CAD build for the part. Positions are in the model's coordinates, mm. A direction names the side the tool comes from. Coordinates: 2 decimals unless noted, no trailing zeros. Loops run counter-clockwise (first coordinate to the right, second up) from the corner with the lowest first, then second, coordinate; pieces in that order, holes last. Notation, with made-up numbers: (70, 34) -> (105, 34) arc R8 ccw to (105, 41) -> close; hole circle Ø4 at (4, 17.5). An arc over 180 degrees is marked (long way). Write each question's results on one line, items separated by ' | '.
```python
from build123d import *

# Parameters (mm, degrees)
SKETCH1_W                     = 60
SKETCH1_H                     = 120
BASE_FLANGE1_DEPTH            = 1.5
CUT_EXTRUDE1_DEPTH            = 10
BREAK_CORNER1_START           = -1.5
BREAK_CORNER1_DEPTH           = 1.5
EDGE_FLANGE1_STRIP_W          = 8
EDGE_FLANGE1_STRIP_H          = 1.5
EDGE_FLANGE1_STRIP_CUT_DEPTH  = 20
EDGE_FLANGE1_RELIEF_W         = 9.5
EDGE_FLANGE1_RELIEF_H         = 1.5
EDGE_FLANGE1_RELIEF_CUT_DEPTH = 1.5
EDGE_FLANGE1_DEPTH            = 20
SKETCH10_R                    = 4
CUT_EXTRUDE2_DEPTH            = 10
MIRROR2_COPY_1_SKETCH_W       = 8
MIRROR2_COPY_1_SKETCH_H       = 1.5
MIRROR2_COPY_1_DEPTH          = 20
MIRROR2_COPY_2_SKETCH_W       = 9.5
MIRROR2_COPY_2_SKETCH_H       = 1.5
MIRROR2_COPY_2_DEPTH          = 1.5
MIRROR2_COPY_3_DEPTH          = 20
MIRROR2_COPY_4_SKETCH_R       = 4
MIRROR2_COPY_4_DEPTH          = 10
BREAK_CORNER2_START           = -30
BREAK_CORNER2_DEPTH           = 60


# Read off the part's stored shape, not the designer's step: Break-Corner1, Break-Corner2
# Sheet-metal steps are written as plain solids
with BuildPart() as part:
    # Sketch1 → Base-Flange1 (new body)
    with BuildSketch(Plane(origin=(0, 0, 0), x_dir=(1, 0, 0), z_dir=(0, 1, 0))):
        Rectangle(SKETCH1_W, SKETCH1_H)
    extrude(amount=-BASE_FLANGE1_DEPTH)

    # Sketch6 → Cut-Extrude1 (cut)
    with BuildSketch(Plane(origin=(0, 0, 0), x_dir=(1, 0, 0), z_dir=(0, 1, 0))):
        with BuildLine():
            Line((18, 30), (18, -30))
            ThreePointArc((18, -30), (0, -48), (-18, -30))
            Line((-18, -30), (-18, 30))
            ThreePointArc((-18, 30), (0, 48), (18, 30))
        make_face()
    extrude(amount=-CUT_EXTRUDE1_DEPTH, mode=Mode.SUBTRACT)

    # Break-Corner1 outline → Break-Corner1 (cut)
    with BuildSketch(Plane(origin=(0, 0, 0), x_dir=(1, 0, 0), z_dir=(0, 1, 0)).offset(BREAK_CORNER1_START)):
        with BuildLine():
            ThreePointArc((30, -50), (27.071067812, -57.071067812), (20, -60))
            Line((20, -60), (30, -60))
            Line((30, -60), (30, -50))
        make_face()
        with BuildLine():
            Line((-30, -60), (-20, -60))
            ThreePointArc((-20, -60), (-27.071067812, -57.071067812), (-30, -50))
            Line((-30, -50), (-30, -60))
        make_face()
        with BuildLine():
            ThreePointArc((20, 60), (27.071067812, 57.071067812), (30, 50))
            Line((30, 50), (30, 60))
            Line((30, 60), (20, 60))
        make_face()
        with BuildLine():
            Line((-30, 60), (-30, 50))
            ThreePointArc((-30, 50), (-27.071067812, 57.071067812), (-20, 60))
            Line((-20, 60), (-30, 60))
        make_face()
    extrude(amount=BREAK_CORNER1_DEPTH, mode=Mode.SUBTRACT)

    # Edge-Flange1 strip (across the edge) → Edge-Flange1 strip cut (cut)
    with BuildSketch(Plane(origin=(30, -1.5, 25), x_dir=(-1, 0, 0), z_dir=(0, 0, 1))):
        with Locations((-1.5, -0.75)):
            Rectangle(EDGE_FLANGE1_STRIP_W, EDGE_FLANGE1_STRIP_H)
    edge_flange1_strip_cut = extrude(amount=EDGE_FLANGE1_STRIP_CUT_DEPTH, mode=Mode.SUBTRACT)

    # Edge-Flange1 relief (on the sheet) → Edge-Flange1 relief cut (cut)
    with BuildSketch(Plane(origin=(27.5, -1.5, 25), x_dir=(-1, 0, 0), z_dir=(0, -1, 0))):
        with Locations((-3.25, 0.75)):
            Rectangle(EDGE_FLANGE1_RELIEF_W, EDGE_FLANGE1_RELIEF_H)
        with Locations((-3.25, -20.75)):
            Rectangle(EDGE_FLANGE1_RELIEF_W, EDGE_FLANGE1_RELIEF_H)
    edge_flange1_relief_cut = extrude(amount=-EDGE_FLANGE1_RELIEF_CUT_DEPTH, mode=Mode.SUBTRACT)

    # Edge-Flange1 section (across the edge) → Edge-Flange1 (add)
    with BuildSketch(Plane(origin=(30, -1.5, 25), x_dir=(-1, 0, 0), z_dir=(0, 0, 1))):
        with BuildLine():
            Line((0, 1), (0, 28.5))
            Line((0, 28.5), (1.5, 28.5))
            Line((1.5, 28.5), (1.5, 1))
            ThreePointArc((1.5, 1), (1.792893219, 0.292893219), (2.5, 0))
            Line((2.5, 0), (2.5, -1.5))
            ThreePointArc((2.5, -1.5), (0.732233047, -0.767766953), (0, 1))
        make_face()
    edge_flange1 = extrude(amount=EDGE_FLANGE1_DEPTH)

    # Sketch10 → Cut-Extrude2 (cut)
    with BuildSketch(Plane(origin=(30, 0, 0), x_dir=(0, 0, -1), z_dir=(1, 0, 0))):
        with Locations(Location((-35, -20, 0), (0, 0, 90))):
            Circle(SKETCH10_R)
    cut_extrude2 = extrude(amount=-CUT_EXTRUDE2_DEPTH, mode=Mode.SUBTRACT)

    # Mirror1: Edge-Flange1 strip cut, Edge-Flange1 relief cut, Edge-Flange1, Cut-Extrude2 across plane
    add(edge_flange1_strip_cut.mirror(Plane.XY), mode=Mode.SUBTRACT)
    add(edge_flange1_relief_cut.mirror(Plane.XY), mode=Mode.SUBTRACT)
    add(edge_flange1.mirror(Plane.XY))
    add(cut_extrude2.mirror(Plane.XY), mode=Mode.SUBTRACT)

    # Mirror2: Edge-Flange1 strip cut, Edge-Flange1 relief cut, Edge-Flange1, Cut-Extrude2 across plane
    add(edge_flange1_strip_cut.mirror(Plane(origin=(0, 0, 0), x_dir=(0, 0, 1), z_dir=(1, 0, 0))), mode=Mode.SUBTRACT)
    add(edge_flange1_relief_cut.mirror(Plane(origin=(0, 0, 0), x_dir=(0, 0, 1), z_dir=(1, 0, 0))), mode=Mode.SUBTRACT)
    add(edge_flange1.mirror(Plane(origin=(0, 0, 0), x_dir=(0, 0, 1), z_dir=(1, 0, 0))))
    add(cut_extrude2.mirror(Plane(origin=(0, 0, 0), x_dir=(0, 0, 1), z_dir=(1, 0, 0))), mode=Mode.SUBTRACT)

    # Mirror2 copy 1 sketch → Mirror2 copy 1 (cut)
    with BuildSketch(Plane(origin=(-30, -1.5, -25), x_dir=(1, 0, 0), z_dir=(0, 0, -1))):
        with Locations((-1.5, -0.75)):
            Rectangle(MIRROR2_COPY_1_SKETCH_W, MIRROR2_COPY_1_SKETCH_H)
    extrude(amount=MIRROR2_COPY_1_DEPTH, mode=Mode.SUBTRACT)

    # Mirror2 copy 2 sketch → Mirror2 copy 2 (cut)
    with BuildSketch(Plane(origin=(-27.5, -1.5, -25), x_dir=(1, 0, 0), z_dir=(0, -1, 0))):
        with Locations((-3.25, 0.75)):
            Rectangle(MIRROR2_COPY_2_SKETCH_W, MIRROR2_COPY_2_SKETCH_H)
        with Locations((-3.25, -20.75)):
            Rectangle(MIRROR2_COPY_2_SKETCH_W, MIRROR2_COPY_2_SKETCH_H)
    extrude(amount=-MIRROR2_COPY_2_DEPTH, mode=Mode.SUBTRACT)

    # Mirror2 copy 3 sketch → Mirror2 copy 3 (add)
    with BuildSketch(Plane(origin=(-30, -1.5, -25), x_dir=(1, 0, 0), z_dir=(0, 0, -1))):
        with BuildLine():
            Line((0, 1), (0, 28.5))
            Line((0, 28.5), (1.5, 28.5))
            Line((1.5, 28.5), (1.5, 1))
            ThreePointArc((1.5, 1), (1.792893219, 0.292893219), (2.5, 0))
            Line((2.5, 0), (2.5, -1.5))
            ThreePointArc((2.5, -1.5), (0.732233047, -0.767766953), (0, 1))
        make_face()
    extrude(amount=MIRROR2_COPY_3_DEPTH)

    # Mirror2 copy 4 sketch → Mirror2 copy 4 (cut)
    with BuildSketch(Plane.ZY.offset(30)):
        with Locations(Location((-35, -20, 0), (0, 0, 90))):
            Circle(MIRROR2_COPY_4_SKETCH_R)
    extrude(amount=-MIRROR2_COPY_4_DEPTH, mode=Mode.SUBTRACT)

    # Break-Corner2 outline → Break-Corner2 (cut)
    with BuildSketch(Plane.YZ.offset(BREAK_CORNER2_START)):
        with BuildLine():
            Line((-30, 45), (-30, 40))
            ThreePointArc((-30, 40), (-28.535533906, 43.535533906), (-25, 45))
            Line((-25, 45), (-30, 45))
        make_face()
        with BuildLine():
            ThreePointArc((-25, 25), (-28.535533906, 26.464466094), (-30, 30))
            Line((-30, 30), (-30, 25))
            Line((-30, 25), (-25, 25))
        make_face()
        with BuildLine():
            ThreePointArc((-25, -45), (-28.535533906, -43.535533906), (-30, -40))
            Line((-30, -40), (-30, -45))
            Line((-30, -45), (-25, -45))
        make_face()
        with BuildLine():
            Line((-30, -25), (-30, -30))
            ThreePointArc((-30, -30), (-28.535533906, -26.464466094), (-25, -25))
            Line((-25, -25), (-30, -25))
        make_face()
    extrude(amount=BREAK_CORNER2_DEPTH, mode=Mode.SUBTRACT)


solid = part.part
```
Q1. Which spindle directions (+Z, -Z, +X, -X, +Y, -Y) get a long thin tool onto all of the face, cutting with end or side? Do faces 1 (the cylindrical face through (29.248, -0.713, -34.86)), 2 (the flat face through (29, -12, 45)), 3 (the flat face through (-29, -12, -45)), 4 (the cylindrical face through (-29.248, -0.713, 34.86)), 5 (the flat face through (28.5, -13, -35)). Say none if no direction does.
Results are:
face 1: +X, +Y | face 2: +X, +Y, -Y | face 3: -X, +Y, -Y | face 4: -X, +Y | face 5: +Z, -Z, -Y
Q2. Drop flat-ended pins along their axis: pin 1 (4.5 mm diameter, centred on x = -28.5, y = -13, fed in from +Z); pin 2 (12 mm diameter, centred on y = -10, z = 15, fed in from +X); pin 3 (0.8 mm diameter, centred on y = -0.5, z = -24, fed in from +X); pin 4 (0.8 mm diameter, centred on x = -28.5, y = -1, fed in from -Z). Give the stop position or say it passes through.
Results are:
pin 1: z = 45 | pin 2: through | pin 3: x = 26 | pin 4: z = -55.86
Q3. Cut at D-D on y = -20. Give the number of separate pieces and of enclosed holes in the cut face, and give its area (3 significant figures).
Results are:
separate pieces: 8 | enclosed holes: 0 | area: 72.0 mm^2
Q4. Wall check: L1, parallel to Z at x = 29.65, y = -20; L2, parallel to X at y = -12.75, z = -27.5; L3, parallel to Y at x = -25, z = 44.5. Give the ranges that are in metal, low to high. Write a range as from..to.
Results are:
L1: -45..-39, -31..-25, 25..31, 39..45 | L2: -30..-28.5, 28.5..30 | L3: -1.5..0
Q5. Pull direction Y, two halves, no side cores. Call faces 6 (the cylindrical face through (-29.26, -20.521, -38.966)), 7 (the cylindrical face through (-29, -28, -44)), 8 (the cylindrical face through (-26.99, -0.76, 57.15)): +Y half, -Y half, draft (parallel to the pull), parting line (faces both ways), or undercut.
Results are:
face 6: undercut | face 7: -Y half | face 8: draft
Q6. Cut at A-A on y = -12.25. Write the cut outline in (x, z).
Results are:
outline: (-30, -45) -> (-28.5, -45) -> (-28.5, -25) -> (-30, -25) -> close; (-30, 25) -> (-28.5, 25) -> (-28.5, 45) -> (-30, 45) -> close; (28.5, -45) -> (30, -45) -> (30, -25) -> (28.5, -25) -> close; (28.5, 25) -> (30, 25) -> (30, 45) -> (28.5, 45) -> close
Q7. Cut at C-C on z = -10. Write the cut outline in (x, y), and give its area (3 significant figures).
Results are:
outline: (-30, -1.5) -> (-18, -1.5) -> (-18, 0) -> (-30, 0) -> close; (18, -1.5) -> (30, -1.5) -> (30, 0) -> (18, 0) -> close | area: 36.0 mm^2
Q8. Cut at B-B on x = 0. Write the cut outline in (y, z), and give its area (3 significant figures).
Results are:
outline: (-1.5, -60) -> (0, -60) -> (0, -48) -> (-1.5, -48) -> close; (-1.5, 48) -> (0, 48) -> (0, 60) -> (-1.5, 60) -> close | area: 36.0 mm^2
